Answer from the drawing. Dimensions are ordinates in mm from the lowest x, y and z of the part. A direction names the side the tool comes from. Coordinates: 2 decimals unless noted, no trailing zeros. Order: outer loops, then holes, each group sorted by start corner. A loop starts at its lowest first (then second) coordinate and runs counter-clockwise, first axis right, second up. Notation, with made-up numbers: (-2.75, 51) -> (21.25, 51) arc R25 cw to (21.25, 78) -> close; hole circle Ø9 at (41.5, 8). An arc over 180 degrees is marked (long way). Use CSV: the item, a comma, the result in double quotes.
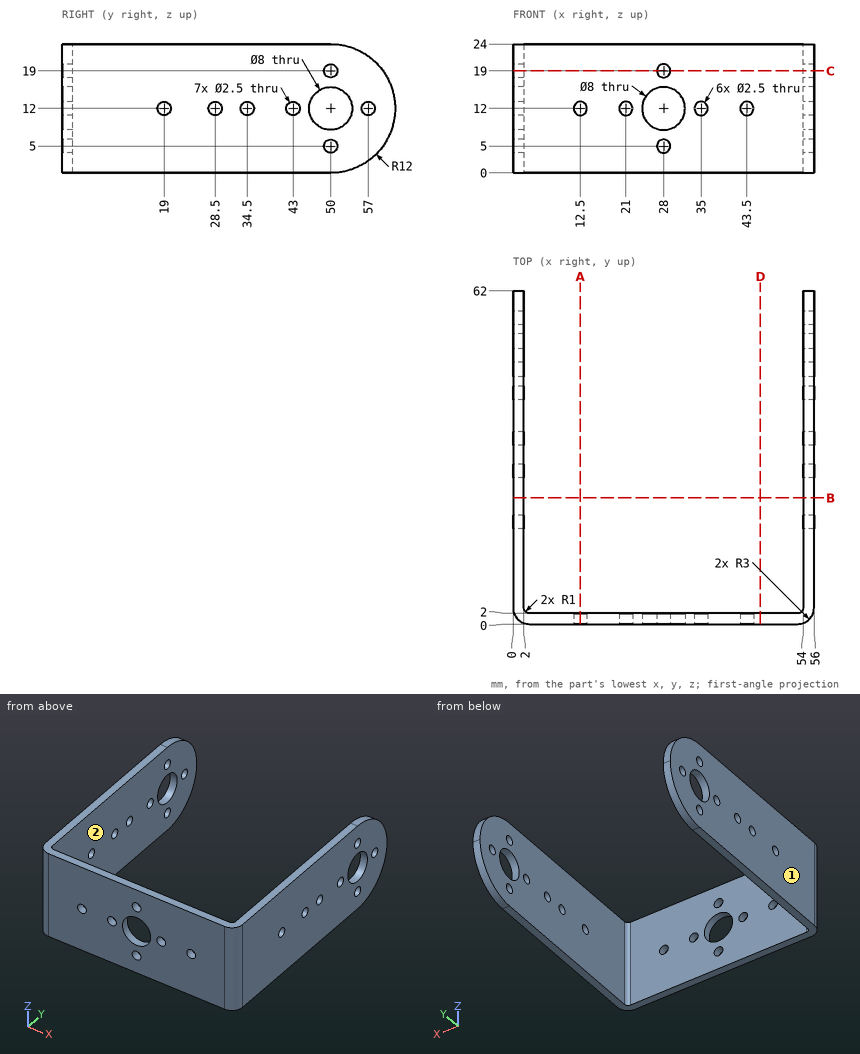
Item 1: Straight lines are drawn through the part: line 1 along Z through (x, y) = (28, 1); line 2 along X through (y, z) = (24, 4.75); line 3 along Y through (x, z) = (55.55, 19). For each, find the intervals that lie inside material, in ascending order.
Return value:
line 1,"z = 0 to 3.75, 6.25 to 8, 16 to 17.75, 20.25 to 24"
line 2,"x = 0 to 2, 54 to 56"
line 3,"y = 1.42 to 48.75, 51.25 to 59.75"
Item 2: Find section B-B, the plane y = 23.5. Give the vertices of the cut face in (x, z), then the cut area to 3 significant figures.
Return value:
outline,"(0, 0) -> (2, 0) -> (2, 24) -> (0, 24) -> close; (54, 0) -> (56, 0) -> (56, 24) -> (54, 24) -> close"
area,"96.0 mm^2"
Item 3: Find section C-C, the plane z = 19. Give the vertices of the cut face in (x, y).
Return value:
outline,"(0, 3) arc R3 ccw to (3, 0) -> (26.75, 0) -> (26.75, 2) -> (3, 2) arc R1 cw to (2, 3) -> (2, 48.75) -> (0, 48.75) -> close; (0, 51.25) -> (2, 51.25) -> (2, 59.75) -> (0, 59.75) -> close; (29.25, 0) -> (53, 0) arc R3 ccw to (56, 3) -> (56, 48.75) -> (54, 48.75) -> (54, 3) arc R1 cw to (53, 2) -> (29.25, 2) -> close; (54, 51.25) -> (56, 51.25) -> (56, 59.75) -> (54, 59.75) -> close"
Item 4: This flat-tipped pin is pushed along its axis until it touches: P1, Ø9, axis at x = 28, z = 12, coming from the +Y side. Where does it stop, or does it pass through?
Return value:
P1,"stops at y = 2"
Item 5: A tool of negligible diameter and unlimited length cuts with its end or side. For the marked faces 1 and 2, from which of +Z, -Z, +X, -X, +Y, -Y can it reach the whole face along a straight path? Write none if from no direction.
Return value:
face 1,"+Z, -Z, -X, +Y, -Y"
face 2,"+Z, -Z, +Y"
Item 6: Find section D-D, the plane x = 46. Give the vertices of the cut face in (y, z), then the cut area to 3 significant figures.
Return value:
outline,"(0, 0) -> (2, 0) -> (2, 24) -> (0, 24) -> close"
area,"48.0 mm^2"
Item 7: Find section A-A, the plane x = 12.5. Give the vertices of the cut face in (y, z), then the cut area to 3 significant figures.
Return value:
outline,"(0, 0) -> (2, 0) -> (2, 10.75) -> (0, 10.75) -> close; (0, 13.25) -> (2, 13.25) -> (2, 24) -> (0, 24) -> close"
area,"43.0 mm^2"
